For this review, take the finished solid that the model builds, in its own axes (mm). Round coordinates to 2 decimals unless told otherwise and drop trailing zeros. Order: outer loops, then holes, each group sorted by start corner. A loop starts at its lowest first (then second) coordinate and runs counter-clockwise, first axis right, second up. Notation, with made-up numbers: M 54.5,88 L 75.5,88 A13 cw 75.5,109 Z; hole C 47,16.25 d3. An arc over 180 degrees is marked long. Use a Markdown table: item, result.
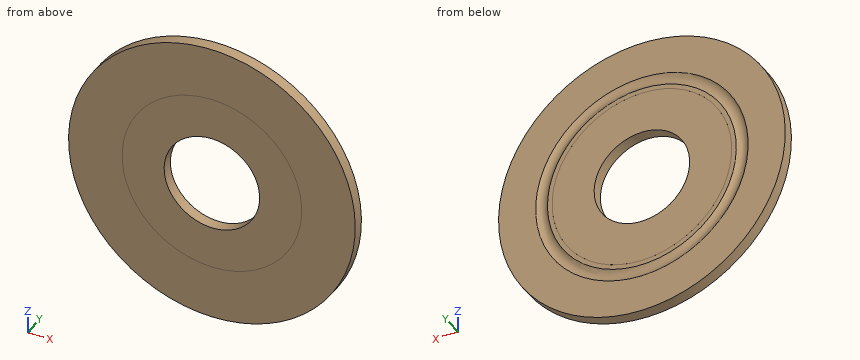
from build123d import *

# Parameters (mm, degrees)
SKETCH2_R           = 75
SKETCH2_R_2         = 59
SKETCH2_R_3         = 46.992946112
BOSS_EXTRUDE1_DEPTH = 6
SKETCH8_R           = 25
CUT_EXTRUDE4_DEPTH  = 6


with BuildPart() as part:
    # Sketch1 → Revolve1 (revolve)
    with BuildSketch(Plane(origin=(0, 0, 0), x_dir=(-1, 0, 0), z_dir=(0, 0, -1)), mode=Mode.PRIVATE) as revolve1_sk:
        with BuildLine():
            Line((-59, 0.8724), (-47, 0.8724))
            ThreePointArc((-47, 0.8724), (-46.292893219, 1.165293219), (-46, 1.8724))
            Line((-46, 1.8724), (-46, 5.8724))
            Line((-46, 5.8724), (-47, 6.8724))
            Line((-47, 6.8724), (-49.4043, 6.8724))
            ThreePointArc((-49.4043, 6.8724), (-52.5, 5.8405), (-55.5957, 6.8724))
            Line((-55.5957, 6.8724), (-59, 6.8724))
            Line((-59, 6.8724), (-60, 5.8724))
            Line((-60, 5.8724), (-60, 1.8724))
            ThreePointArc((-60, 1.8724), (-59.707106781, 1.165293219), (-59, 0.8724))
        make_face()
    revolve(revolve1_sk.sketch.rotate(Axis((0, 0, 0), (0, 1, 0)), 270), axis=Axis((0, 0, 0), (0, 1, 0)))

    # Sketch2 → Boss-Extrude1 (add)
    # profile 1 of 2: a face of its own
    with BuildSketch(Plane.XZ.offset(-0.8724)):
        with Locations(Location((0, 0, 0), (0, 0, 270))):
            Circle(SKETCH2_R)
        Circle(SKETCH2_R_2, mode=Mode.SUBTRACT)
    # profile 2 of 2: a face of its own
    with BuildSketch(Plane.XZ.offset(-0.8724)):
        with Locations(Location((0, 0, 0), (0, 0, 270))):
            Circle(SKETCH2_R_3)
    extrude(amount=-BOSS_EXTRUDE1_DEPTH)

    # Sketch8 → Cut-Extrude4 (cut)
    with BuildSketch(Plane(origin=(0, 6.8724, 0), x_dir=(1, 0, 0), z_dir=(0, 1, 0))):
        with Locations(Location((0, 0, 0), (0, 0, 270))):
            Circle(SKETCH8_R)
    extrude(amount=-CUT_EXTRUDE4_DEPTH, mode=Mode.SUBTRACT)


solid = part.part
Q1. Clearance check with flat-ended pins moving along their axes: pin 1 (1 mm diameter, centred on y = 2, z = 55.5, fed in from +X); pin 2 (1 mm diameter, centred on x = 21.5, y = 6, fed in from +Z). State where each tip first meets the part, or that it passes through.
Determined:
| item | result |
|---|---|
| pin 1 | stops at x = 50.99 |
| pin 2 | stops at z = 72 |
Q2. Add section C-C (y = 2.75). Write out the cut boundary in (x, z), then the cut area to 3 significant figures.
Determined:
| item | result |
|---|---|
| outline | C 0,0 d150; hole C 0,0 d50 |
| area | 15,700 mm^2 |
Q3. Add section D-D (z = 63.5). Write out the cut boundary in (x, y).
Determined:
| item | result |
|---|---|
| outline | M -39.91,0.87 L 39.91,0.87 L 39.91,6.87 L -39.91,6.87 Z |
Q4. Wall thickness on line 1 along X through (y, z) = (2.3, 0); line 2 along X through (y, z) = (6.5, -26.5); line 3 along Y through (x, z) = (-9.5, -51): over which ranges is each line inside the solid? List them lowest first. Write a range as [from, to].
Determined:
| item | result |
|---|---|
| line 1 | x = [-75, -25], [25, 75] |
| line 2 | x = [-70.16, -48.22], [-42.37, 42.37], [48.22, 70.16] |
| line 3 | y = [0.87, 5.88] |
